```python
from build123d import *

# Parameters (mm, degrees)
SKETCH2_W                   = 46.5
SKETCH2_H                   = 97.9
SKETCH2_W_2                 = 32.3
SKETCH2_H_2                 = 83.05
BOSS_EXTRUDE1_DEPTH         = 5
SKETCH2_4_W                 = 32.3
SKETCH2_4_H                 = 83.05
SKETCH2_4_W_2               = 25.4
SKETCH2_4_H_2               = 76.2
BOSS_EXTRUDE2_DEPTH         = 5
TAP_DRILL_FOR_M3X0_5_TAP1_D = 3.75
SKETCH7_R                   = 3.475
SKETCH7_R_2                 = 1.875
BOSS_EXTRUDE5_DEPTH         = 15
BOSS_EXTRUDE4_DEPTH         = 97.55
CUT_EXTRUDE1_DEPTH          = 112.426738894
CUT_EXTRUDE1_DEPTH_BACK     = 112.426738894
CUT_EXTRUDE2_DEPTH          = 100.18712429
CUT_EXTRUDE2_DEPTH_BACK     = 5
SKETCH11_W                  = 10
SKETCH11_H                  = 15
SKETCH12_W                  = 4
SKETCH12_H                  = 8
CUT_EXTRUDE3_DEPTH          = 100.18712429


with BuildPart() as part:
    # Sketch2 → Boss-Extrude1 (new, symmetric)
    with BuildSketch(Plane.XY):
        with Locations((16.15, 41.525)):
            Rectangle(SKETCH2_W, SKETCH2_H)
        with Locations((16.15, 41.525)):
            Rectangle(SKETCH2_W_2, SKETCH2_H_2, mode=Mode.SUBTRACT)
    extrude(amount=BOSS_EXTRUDE1_DEPTH, both=True)

    # Sketch2<4> → Boss-Extrude2 (add)
    # profile 1 of 2: a face of its own
    with BuildSketch(Plane.XY):
        with Locations((16.15, 41.525)):
            Rectangle(SKETCH2_4_W, SKETCH2_4_H)
        with Locations((16.15, 41.525)):
            Rectangle(SKETCH2_4_W_2, SKETCH2_4_H_2, mode=Mode.SUBTRACT)
    # profile 2 of 2: a face of its own
    with BuildSketch(Plane.XY):
        with Locations((16.15, 41.525)):
            Rectangle(SKETCH2_4_W_2, SKETCH2_4_H_2)
    extrude(amount=-BOSS_EXTRUDE2_DEPTH)

    # Tap Drill for M3x0.5 Tap1 (through all)
    with Locations(Plane.XY):
        with Locations((3.45, 79.625), (28.85, 79.625), (3.45, 3.425), (28.85, 3.425)):
            Hole(TAP_DRILL_FOR_M3X0_5_TAP1_D / 2)

    # Sketch7 → Boss-Extrude5 (add)
    # profile 1 of 4: a face of its own
    with BuildSketch(Plane.XY):
        with Locations((-3.225, 86.525)):
            Circle(SKETCH7_R)
        with Locations((-3.225, 86.525)):
            Circle(SKETCH7_R_2, mode=Mode.SUBTRACT)
    # profile 2 of 4: a face of its own
    with BuildSketch(Plane.XY):
        with Locations((35.525, 86.525)):
            Circle(SKETCH7_R)
        with Locations((35.525, 86.525)):
            Circle(SKETCH7_R_2, mode=Mode.SUBTRACT)
    # profile 3 of 4: a face of its own
    with BuildSketch(Plane.XY):
        with Locations((-3.225, -3.475)):
            Circle(SKETCH7_R)
        with Locations((-3.225, -3.475)):
            Circle(SKETCH7_R_2, mode=Mode.SUBTRACT)
    # profile 4 of 4: a face of its own
    with BuildSketch(Plane.XY):
        with Locations((35.525, -3.475)):
            Circle(SKETCH7_R)
        with Locations((35.525, -3.475)):
            Circle(SKETCH7_R_2, mode=Mode.SUBTRACT)
    extrude(amount=BOSS_EXTRUDE5_DEPTH)

    # Sketch11 → Cut-Extrude2 (cut, two sides: drawn at the far end of the back side and taken through both)
    with BuildSketch(Plane.XY.offset(5).offset(-CUT_EXTRUDE2_DEPTH_BACK)):
        with Locations((16.15, 83.05)):
            Rectangle(SKETCH11_W, SKETCH11_H)
    extrude(amount=CUT_EXTRUDE2_DEPTH + CUT_EXTRUDE2_DEPTH_BACK, mode=Mode.SUBTRACT)

    # Sketch12 → Cut-Extrude3 (cut, through all)
    with BuildSketch(Plane.XY.offset(5)):
        with Locations((16.15, -7.425)):
            Rectangle(SKETCH12_W, SKETCH12_H)
    extrude(amount=-CUT_EXTRUDE3_DEPTH, mode=Mode.SUBTRACT)


with BuildPart() as body_2:
    # Sketch6 → Boss-Extrude4 (new body)
    with BuildSketch(Plane(origin=(0, 90.475, 0), x_dir=(1, 0, 0), z_dir=(0, 1, 0))):
        with BuildLine():
            Line((-12.283937642, -5.441846212), (-12.33484351, -5.441846212))
            ThreePointArc((-12.33484351, -5.441846212), (16.097911959, -28.999953221), (44.615111123, -5.544136432))
            Line((44.615111123, -5.544136432), (44.564169902, -5.544136432))
            ThreePointArc((44.564169902, -5.544136432), (16.097908608, -28.949953134), (-12.283937642, -5.441846212))
        make_face()
    extrude(amount=-BOSS_EXTRUDE4_DEPTH)

    # Sketch6<2> → Cut-Extrude1 (cut, two sides: drawn at the far end of the back side and taken through both)
    with BuildSketch(Plane(origin=(0, 90.475, 0), x_dir=(1, 0, 0), z_dir=(0, 1, 0)).offset(-CUT_EXTRUDE1_DEPTH_BACK)):
        with BuildLine():
            Line((-12.283937642, -5.441846212), (-12.33484351, -5.441846212))
            ThreePointArc((-12.33484351, -5.441846212), (16.097911959, -28.999953221), (44.615111123, -5.544136432))
            Line((44.615111123, -5.544136432), (44.564169902, -5.544136432))
            ThreePointArc((44.564169902, -5.544136432), (16.097908608, -28.949953134), (-12.283937642, -5.441846212))
        make_face()
    extrude(amount=CUT_EXTRUDE1_DEPTH + CUT_EXTRUDE1_DEPTH_BACK, mode=Mode.SUBTRACT)


solid = part.part
```
The model under review builds one solid part; all positions refer to its coordinate system, in mm. A direction names the side the tool comes from. Give positions to 0.01 mm unless a question says otherwise; leave off trailing zeros. Write each loop counter-clockwise with the first axis right and the second up, starting at its lowest first coordinate (ties: lowest second). Pieces come first, ordered by that corner, then holes. Notation, with made-up numbers: (24, -14) - (46, -14) arc R16 cw to (46, 15) - close; hole circle Ø11 at (54, 38). An arc over 180 degrees is marked (long way). Answer in a Markdown table with one row per item. Add a question column.
1. Wall thickness on line 1 along Y through (x, z) = (3.45, -1.1) (3 decimals); line 2 along X through (y, z) = (85.5, 8.75); line 3 along X through (y, z) = (13.5, 0.75): over which ranges is each line inside the solid? List them lowest first. Write a range as [from, to].
2. We need section D-D on x = 25.5. Write out the cut boundary in (y, z) (3 decimals).
3. We need section C-C on y = 66. Write out the cut boundary in (x, z).
4. We need section B-B on z = 9.25. Write out the cut boundary in (x, y) (3 decimals).
5. Tool access review of faces 1 (the flat face through (21.15, 87, 2)), 2 (the flat face through (35, 87, 5)), 3 (the cylindrical face through (3.694, 5.284, -2.535)), 4 (the flat face through (14.15, -5, 0)): name each direction out of +Z, -Z, +X, -X, +Y, -Y from which nothing blocks a thin tool from reaching the whole face with its end or side.
6. Draft analysis for pull direction Y (two halves, no side actions). For faces 5 (the cylindrical face through (33.65, -3.39, 9.93)), 6 (the flat face through (16, 90.475, -1)), 7 (the flat face through (37, 85, 15)), state which applies: +Y half, -Y half, draft (parallel to the pull), parting line (faces both ways), or undercut.
7. We need section A-A on x = 3.45. Write out the cut boundary in (y, z) (3 decimals).
8. Insertion check: P1, Ø3.5, axis at x = -3.225, y = -3.475, coming from the +Z side; P2, Ø10, axis at x = 17, z = 7.5, coming from the +Y side (3 decimals); P3, Ø6, axis at x = 28, y = 59, coming from the +Z side. Each pin has a flat end and moves straight along its axis. Give the tip position at first contact, or say it passes through.
Ans:
| question | item | result |
|---|---|---|
| 1 | line 1 | y = [-7.425, 1.55], [5.3, 77.75], [81.5, 90.475] |
| 1 | line 2 | x = [-6.55, -4.8], [-1.65, 0.1], [32.2, 33.95], [37.1, 38.85] |
| 1 | line 3 | x = [-7.1, 0], [32.3, 39.4] |
| 2 | outline | (-7.425, -5) - (90.475, -5) - (90.475, 5) - (83.05, 5) - (83.05, 0) - (0, 0) - (0, 5) - (-7.425, 5) - close |
| 3 | outline | (-7.1, -5) - (39.4, -5) - (39.4, 5) - (32.3, 5) - (32.3, 0) - (0, 0) - (0, 5) - (-7.1, 5) - close |
| 4 | outline | circle Ø6.95 at (-3.225, -3.475); circle Ø6.95 at (-3.225, 86.525); circle Ø6.95 at (35.525, -3.475); circle Ø6.95 at (35.525, 86.525); hole circle Ø3.75 at (-3.225, -3.475); hole circle Ø3.75 at (-3.225, 86.525); hole circle Ø3.75 at (35.525, -3.475); hole circle Ø3.75 at (35.525, 86.525) |
| 5 | face 1 | +Z, +Y |
| 5 | face 2 | +Z |
| 5 | face 3 | +Z, -Z |
| 5 | face 4 | +Z, -Z, -Y |
| 6 | face 5 | undercut |
| 6 | face 6 | +Y half |
| 6 | face 7 | draft |
| 7 | outline | (-7.425, -5) - (1.55, -5) - (1.55, 0) - (0, 0) - (0, 5) - (-7.425, 5) - close; (5.3, -5) - (77.75, -5) - (77.75, 0) - (5.3, 0) - close; (81.5, -5) - (90.475, -5) - (90.475, 5) - (83.05, 5) - (83.05, 0) - (81.5, 0) - close |
| 8 | P1 | stops at z = 5 |
| 8 | P2 | stops at y = 90.475 |
| 8 | P3 | stops at z = 0 |
